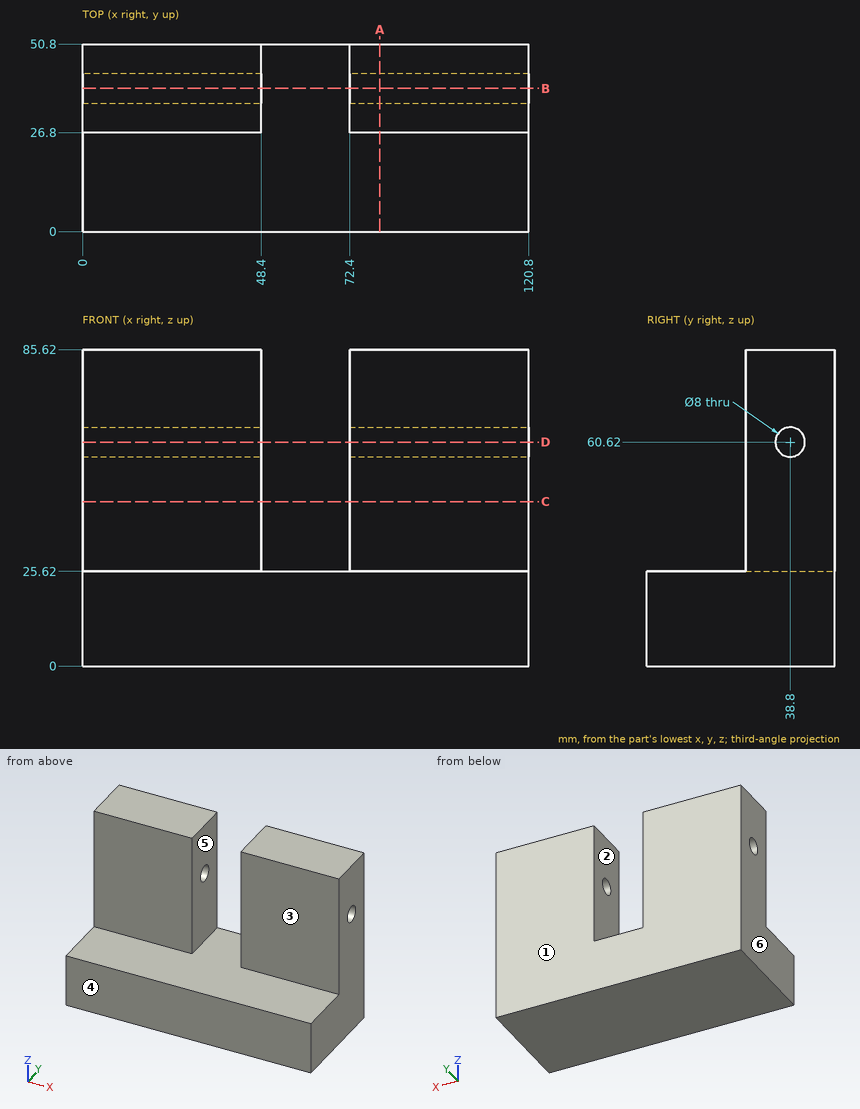
For this review, use the dimensioned drawing (mm, ordinates from the lowest corner) and the shaded views. A direction names the side the tool comes from. Round coordinates to 2 decimals unless told otherwise and drop trailing zeros. Write each loop counter-clockwise with the first axis right and the second up, starting at its lowest first coordinate (ties: lowest second). Pieces come first, ordered by that corner, then holes. Notation, with made-up numbers: (-20.5, -22) -> (14.5, -22) arc R23 ccw to (14.5, -8) -> close; hole circle Ø7 at (37.25, 75.5). An arc over 180 degrees is marked (long way). Use CSV: the item, a comma, the result in double quotes.
(1) For the marked faces 1, 2 and 3, list the 3-axis set-ups (+Z, -Z, +X, -X, +Y, -Y) from which the entire face can be reached by the end or side of a thin tool; tool diameter is ignored.
Computed values:
face 1,"+Z, -Z, +X, -X, +Y"
face 2,"+Z, +Y, -Y"
face 3,"+Z, +X, -X, -Y"
(2) Consider section D-D, the plane z = 60.62. Give the boundary of the cut face in (x, y), plus the area to 3 significant figures.
Computed values:
outline,"(0, 26.8) -> (48.4, 26.8) -> (48.4, 34.8) -> (0, 34.8) -> close; (0, 42.8) -> (48.4, 42.8) -> (48.4, 50.8) -> (0, 50.8) -> close; (72.4, 26.8) -> (120.8, 26.8) -> (120.8, 34.8) -> (72.4, 34.8) -> close; (72.4, 42.8) -> (120.8, 42.8) -> (120.8, 50.8) -> (72.4, 50.8) -> close"
area,"1,550 mm²"
(3) Consider section A-A, the plane x = 80.5. Give the boundary of the cut face in (y, z).
Computed values:
outline,"(0, 0) -> (50.8, 0) -> (50.8, 85.62) -> (26.8, 85.62) -> (26.8, 25.62) -> (0, 25.62) -> close; hole circle Ø8 at (38.8, 60.62)"
(4) Clearance check with flat-ended pins moving along their axes: P1, Ø7, axis at y = 38.8, z = 60.62, coming from the +X side; P2, Ø8, axis at x = 24.5, z = 44.5, coming from the -Y side; P3, Ø8, axis at x = 60.5, y = 42.5, coming from the +Z side. State where each tip first meets the part, or that it passes through.
Computed values:
P1,"through"
P2,"y = 26.8"
P3,"z = 25.62"
(5) Draft analysis for pull direction X (two halves, no side actions). For the marked faces 4, 5 and 6, state which applies: +X half, -X half, draft (parallel to the pull), parting line (faces both ways), or undercut.
Computed values:
face 4,"draft"
face 5,"undercut"
face 6,"-X half"
(6) To check wall thickness, follow L1, parallel to X at y = 30, z = 61; L2, parallel to Z at x = 105, y = 38.8; L3, parallel to Z at x = 101, y = 22.5. State the ranges of each line that lie inside material, in increasing order. Write a range as [from, to].
Computed values:
L1,"[0, 48.4], [72.4, 120.8]"
L2,"[0, 56.62], [64.62, 85.62]"
L3,"[0, 25.62]"
(7) Consider section C-C, the plane z = 44.5. Give the boundary of the cut face in (x, y).
Computed values:
outline,"(0, 26.8) -> (48.4, 26.8) -> (48.4, 50.8) -> (0, 50.8) -> close; (72.4, 26.8) -> (120.8, 26.8) -> (120.8, 50.8) -> (72.4, 50.8) -> close"
(8) Consider section B-B, the plane y = 38.8. Give the boundary of the cut face in (x, z), plus the area to 3 significant figures.
Computed values:
outline,"(0, 0) -> (120.8, 0) -> (120.8, 56.62) -> (72.4, 56.62) -> (72.4, 25.62) -> (48.4, 25.62) -> (48.4, 56.62) -> (0, 56.62) -> close; (0, 64.62) -> (48.4, 64.62) -> (48.4, 85.62) -> (0, 85.62) -> close; (72.4, 64.62) -> (120.8, 64.62) -> (120.8, 85.62) -> (72.4, 85.62) -> close"
area,"8,130 mm²"
